Model file for the job. Use its own axes, mm. Face numbers are marked on the shaded views. A direction names the side the tool comes from. Coordinates: 2 decimals unless noted, no trailing zeros. Write each loop counter-clockwise with the first axis right and the second up, starting at its lowest first coordinate (ties: lowest second). Pieces come first, ordered by that corner, then holes.
Q1. Band-saw the part on B-B, the plane x = 0. Write the cut outline in (y, z).
Q2. Band-saw the part on A-A, the plane z = 0. Write the cut outline in (x, y).
Q3. Which spindle directions (+Z, -Z, +X, -X, +Y, -Y) get a long thin tool onto all of the face, cutting with end or side? Do the marked faces 1 and 2. Say none if no direction does.
Q4. Drill centre lines: probe 1 along Y at (x, z) = (8, -7); probe 2 along Y at (x, z) = (17, -10.5); probe 3 along Z at (x, y) = (1, 94). Where is each one in solid material? Low to high.
Q5. Pin check, flat tips, straight feed: P1, Ø1.5, axis at x = 1.5, z = 18, coming from the +Y side; P2, Ø8, axis at x = 6, y = 92.5, coming from the -Z side; P3, Ø10.5, axis at x = 2.5, z = 6.5, coming from the +Y side; P4, Ø4, axis at y = 97.5, z = -10.5, coming from the -X side. Stop position of each tip, or through.
Q6. Band-saw the part on D-D, the plane y = 18. Write the cut outline in (x, z), plus the area to 3 significant figures.
Q7. Band-saw the part on C-C, the plane y = 120. Write the cut outline in (x, z).
from build123d import *

# Parameters (mm, degrees)
F0_R      = 25.5
F1_DEPTH  = 84.92
F2_R      = 21.74
F3_DEPTH  = 14.52
F4_R      = 17.9
F5_DEPTH  = 12.4
F6_R      = 15.09
F7_DEPTH  = 12.5
F8_R      = 9.96
F9_DEPTH  = 16.46
F10_R     = 6.227418
F11_DEPTH = 11.7


with BuildPart() as f1:
    # F0 (on Front) → F1 (new body)
    with BuildSketch(Plane.XZ):
        Circle(F0_R)
    extrude(amount=-F1_DEPTH)

    # F2 (on face) → F3 (join)
    with BuildSketch(Plane(origin=(0, 84.92, 0), x_dir=(-1, 0, 0), z_dir=(0, 1, 0))):
        Circle(F2_R)
    extrude(amount=F3_DEPTH)

    # F4 (on face) → F5 (join)
    with BuildSketch(Plane(origin=(0, 99.44, 0), x_dir=(-1, 0, 0), z_dir=(0, 1, 0))):
        Circle(F4_R)
    extrude(amount=F5_DEPTH)

    # F6 (on face) → F7 (join)
    with BuildSketch(Plane(origin=(0, 111.84, 0), x_dir=(-1, 0, 0), z_dir=(0, 1, 0))):
        Circle(F6_R)
    extrude(amount=F7_DEPTH)

    # F8 (on face) → F9 (join)
    with BuildSketch(Plane(origin=(0, 124.34, 0), x_dir=(-1, 0, 0), z_dir=(0, 1, 0))):
        Circle(F8_R)
    extrude(amount=F9_DEPTH)

    # F10 (on face) → F11 (join)
    with BuildSketch(Plane(origin=(0, 140.8, 0), x_dir=(-1, 0, 0), z_dir=(0, 1, 0))):
        Circle(F10_R)
    extrude(amount=F11_DEPTH)


solid = f1.part
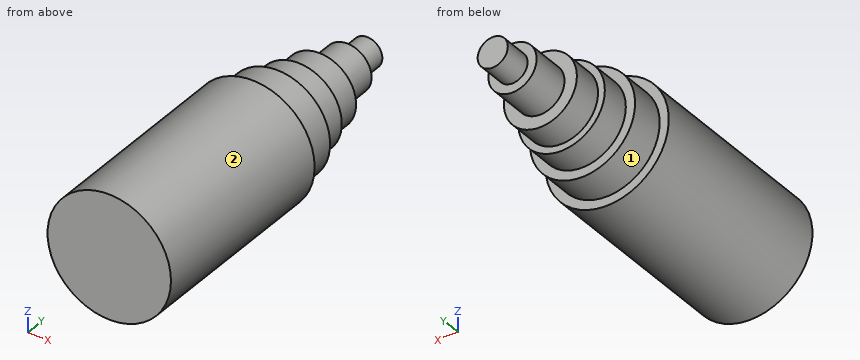
Answer sheet:
1. outline: (0, -25.5) - (84.92, -25.5) - (84.92, -21.74) - (99.44, -21.74) - (99.44, -17.9) - (111.84, -17.9) - (111.84, -15.09) - (124.34, -15.09) - (124.34, -9.96) - (140.8, -9.96) - (140.8, -6.23) - (152.5, -6.23) - (152.5, 6.23) - (140.8, 6.23) - (140.8, 9.96) - (124.34, 9.96) - (124.34, 15.09) - (111.84, 15.09) - (111.84, 17.9) - (99.44, 17.9) - (99.44, 21.74) - (84.92, 21.74) - (84.92, 25.5) - (0, 25.5) - close
2. outline: (-25.5, 0) - (25.5, 0) - (25.5, 84.92) - (21.74, 84.92) - (21.74, 99.44) - (17.9, 99.44) - (17.9, 111.84) - (15.09, 111.84) - (15.09, 124.34) - (9.96, 124.34) - (9.96, 140.8) - (6.23, 140.8) - (6.23, 152.5) - (-6.23, 152.5) - (-6.23, 140.8) - (-9.96, 140.8) - (-9.96, 124.34) - (-15.09, 124.34) - (-15.09, 111.84) - (-17.9, 111.84) - (-17.9, 99.44) - (-21.74, 99.44) - (-21.74, 84.92) - (-25.5, 84.92) - close
3. face 1: +Y
3. face 2: +Y, -Y
4. probe 1: y = 0 to 124.34
4. probe 2: y = 0 to 99.44
4. probe 3: z = -21.72 to 21.72
5. P1: stops at y = 111.84
5. P2: stops at z = -21.65
5. P3: stops at y = 152.5
5. P4: stops at x = -20.01
6. outline: circle Ø51 at (0, 0)
6. area: 2,040 mm2
7. outline: circle Ø30.18 at (0, 0)
